The listing builds one solid part. Answer for the finished solid, in the listing's coordinates (mm). A direction names the side the tool comes from. Give positions to 0.01 mm unless a question says otherwise; leave off trailing zeros. Write each loop counter-clockwise with the first axis right and the second up, starting at its lowest first coordinate (ties: lowest second). Pieces come first, ordered by that corner, then holes. Notation, with made-up numbers: (82.25, 60) -> (137.25, 60) arc R15 cw to (137.25, 77) -> close; hole circle Ø1 at (2.25, 88.5). An arc over 180 degrees is marked (long way). Write each question's results on one line, items separated by ' | '. Start each with the question number.
Autodesk Inventor part; units mm, degrees
ref_plane "YZ Plane" through (0, 0, 0) normal (1, 0, 0) x (0, 1, 0)
ref_plane "XZ Plane" through (0, 0, 0) normal (0, 1, 0) x (-1, 0, 0)
ref_plane "XY Plane" through (0, 0, 0) normal (0, 0, 1) x (1, 0, 0)
sketch "Esquisse1" plane through (0, 0, 0) normal (0, 1, 0) x (-1, 0, 0)
  line L0 (-25.5, 23) -> (-22.5, 23)
  line L1 (-22.5, 23) -> (-22.5, -47)
  line L2 (-22.5, -47) -> (-25.5, -47)
  line L3 (-25.5, -47) -> (-25.5, 23)
  line L4 (-22.5, 23) -> (27.5, 23)
  line L5 (27.5, 23) -> (27.5, 20)
  line L6 (27.5, 20) -> (-22.5, 20)
  line L7 (-22.5, 20) -> (-22.5, 23)
  line L8 (27.5, 20) -> (22.5, 20)
  line L9 (22.5, 20) -> (22.5, -20)
  line L10 (22.5, -20) -> (27.5, -20)
  line L11 (27.5, -20) -> (27.5, 20)
  point P0 (0, 0)
  dimension "d0" = 45
  dimension "d1" = 5
  dimension "d2" = 3
  dimension "d3" = 3
  dimension "d4" = 40
  dimension "d5" = 20
  dimension "d6" = 22.5
  dimension "d7" = 70
extrude "Extrusion1" add sketch "Esquisse1" along normal blind 25
sketch "Esquisse2" plane through (25.5, 0, 23) normal (1, 0, 0) x (0, 0, -1)
  line L0 (70, 0) -> (70, 25)
  line L1 (0, 25) -> (70, 25)
  line L2 (70, 25) -> (63.6, 25)
  line L3 (63.6, 25) -> (63.6, 4)
  line L4 (63.6, 4) -> (70, 4)
  line L5 (70, 4) -> (70, 25)
  line L6 (63.6, 4) -> (21.6, 4)
  line L7 (21.6, 4) -> (21.6, 25)
  line L8 (21.6, 25) -> (63.6, 25)
  line L9 (63.6, 25) -> (63.6, 4)
  line L10 (21.6, 4) -> (15.2, 4)
  line L11 (15.2, 4) -> (15.2, 25)
  line L12 (15.2, 25) -> (21.6, 25)
  line L13 (21.6, 25) -> (21.6, 4)
  line L14 (15.2, 14.5) -> (70, 14.5) construction
  circle A0 centre (18.4, 19.5) radius 2.5
  circle A1 centre (66.8, 19.5) radius 2.5
  circle A2 centre (18.4, 9.5) radius 2.5
  circle A3 centre (66.8, 9.5) radius 2.5
  point P0 (23, 0)
  dimension "d10" = 21
  dimension "d11" = 6.4
  dimension "d12" = 6.4
  dimension "d13" = 42
  dimension "d14" = 5
  dimension "d15" = 5
  dimension "d16" = 5
  dimension "d17" = 3.2
  dimension "d18" = 3.2
  dimension "d19" = 5
sketch "Esquisse3" plane through (25.5, 0, 23) normal (1, 0, 0) x (0, 0, -1)
  line L0 (0, 25) -> (70, 25)
  line L1 (21.6, 4) -> (63.6, 4)
  line L2 (63.6, 4) -> (63.6, 25)
  line L3 (63.6, 25) -> (21.6, 25)
  line L4 (21.6, 25) -> (21.6, 4)
  line L5 (63.6, 4) -> (70, 4)
  line L6 (70, 4) -> (70, 25)
  line L7 (70, 25) -> (63.6, 25)
  line L8 (63.6, 25) -> (63.6, 4)
  line L9 (21.6, 14.5) -> (63.6, 14.5) construction
  circle A0 centre (31.6, 14.5) radius 3.5
  point P0 (23, 0)
  dimension "d22" = 6.4
  dimension "d23" = 21
  dimension "d24" = 42
  dimension "d25" = 7
  dimension "d27" = 10
extrude "Extrusion3" cut sketch "Esquisse3" against normal through all contours A0
extrude "Extrusion4" cut sketch "Esquisse2" against normal up to surface (3 mm away) contours L6 L7 L1 L3 | A0 | A1 | A2 | A3
equation "\"d12\" = d11"
equation "\"d15\" = d14"
equation "\"d18\" = d17"
equation "\"d19\" = d16"
properties part number "new_shoulder_2_modif"
1. The mould has two halves that part along Y. Classify faces 1 (the cylindrical face through (24, 8, -41.8)), 2 (the flat face through (24, 25, -44)), 3 (the flat face through (-22.5, 12, 0)): pulls with the +Y half, pulls with the -Y half, needs draft (parallel to the pull), parting line crosses it, or undercut.
2. Section B-B (z = -8.6) is taken. Write down the section's boundary in (x, y).
3. A tool of negligible diameter and unlimited length cuts with its end or side. For faces 4 (the cylindrical face through (24.02, 7.06, 5.14)), 5 (the flat face through (22.5, 9.5, 1.9)), 6 (the flat face through (24, 15, -40.6)), 7 (the flat face through (24, 14, 1.4)), from which of +Z, -Z, +X, -X, +Y, -Y can it reach the whole face along a straight path? Write none if from no direction.
4. Section A-A (y = 9.5) is taken. Write down the section's boundary in (x, z), then the cut area to 3 significant figures.
5. Each of these flat-tipped pins is pushed along its axis until it touches: pin 1 Ø6.5 at (y, z) = (9.5, -43.8) entering from -X; pin 2 Ø1.5 at (x, y) = (5.5, 3) entering from -Z; pin 3 Ø7.5 at (y, z) = (8.5, -2.5) entering from +X. Where does it stop, or does it pass through?
6. Section D-D (z = 15) is taken. Write down the section's boundary in (x, y).
7. Consider probe 1 along Y at (x, z) = (-25.25, -8.6); probe 2 along Y at (x, z) = (24.7, -43.8); probe 3 along Y at (x, z) = (24, 4). Determine where each line is inside the solid, lowest interval first. Write a range as [from, to].
8. Section C-C (z = 4.6) is taken. Write down the section's boundary in (x, y), then the cut area to 3 significant figures.
Results:
1) face 1: undercut | face 2: pulls with the +Y half | face 3: needs draft
2) outline: (-27.5, 0) -> (-22.5, 0) -> (-22.5, 11) -> (-27.5, 11) -> close; (-27.5, 18) -> (-22.5, 18) -> (-22.5, 25) -> (-27.5, 25) -> close; (22.5, 0) -> (25.5, 0) -> (25.5, 4) -> (22.5, 4) -> close
3) face 4: +X | face 5: -Z, +Y, -Y | face 6: +X, -X, +Y | face 7: +X, +Y
4) outline: (-27.5, -20) -> (-22.5, -20) -> (-22.5, 20) -> (22.5, 20) -> (22.5, 7.1) -> (25.5, 7.1) -> (25.5, 23) -> (-27.5, 23) -> close; (22.5, -47) -> (25.5, -47) -> (25.5, -46.3) -> (22.5, -46.3) -> close; (22.5, -41.3) -> (25.5, -41.3) -> (25.5, -40.6) -> (22.5, -40.6) -> close; (22.5, 1.4) -> (25.5, 1.4) -> (25.5, 2.1) -> (22.5, 2.1) -> close | area: 404 mm²
5) pin 1: stops at x = 22.5 | pin 2: stops at z = 20 | pin 3: stops at x = -22.5
6) outline: (-27.5, 0) -> (-22.5, 0) -> (-22.5, 25) -> (-27.5, 25) -> close; (22.5, 0) -> (25.5, 0) -> (25.5, 25) -> (22.5, 25) -> close
7) probe 1: y = [0, 11], [18, 25] | probe 2: y = [0, 7], [12, 17], [22, 25] | probe 3: y = [0, 7.07], [11.93, 17.07], [21.93, 25]
8) outline: (-27.5, 0) -> (-22.5, 0) -> (-22.5, 25) -> (-27.5, 25) -> close; (22.5, 0) -> (25.5, 0) -> (25.5, 7) -> (22.5, 7) -> close; (22.5, 12) -> (25.5, 12) -> (25.5, 17) -> (22.5, 17) -> close; (22.5, 22) -> (25.5, 22) -> (25.5, 25) -> (22.5, 25) -> close | area: 170 mm²
